For this review, take the finished solid that the model builds, in its own axes (mm). Face numbers are marked on the shaded views. A direction names the side the tool comes from. Coordinates: 2 decimals unless noted, no trailing zeros. Loops run counter-clockwise (first coordinate to the right, second up) from the corner with the lowest first, then second, coordinate; pieces in that order, holes last. Notation, with made-up numbers: M -38.75,19.5 L -9.75,19.5 A4 ccw -9.75,25.5 Z; hole C 62.25,21 d2. An arc over 180 degrees is marked long. Write item = value, one per line.
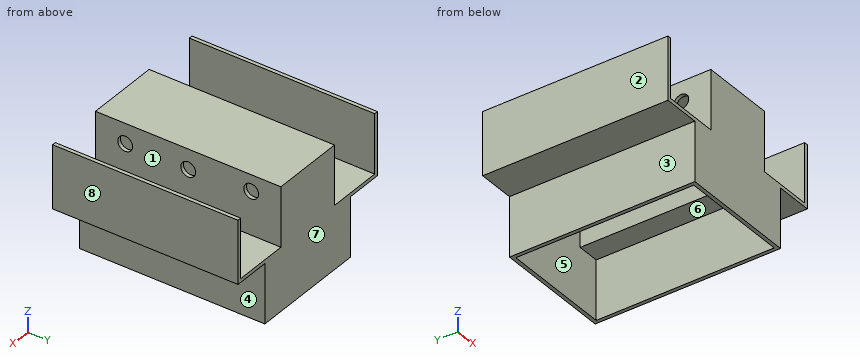
from build123d import *

# Parameters (mm, degrees)
ESQUISSE1_W             = 45
ESQUISSE1_H             = 250
BOSS_EXTRU_1_DEPTH      = 5
ESQUISSE2_W             = 80
ESQUISSE2_H             = 250
BOSS_EXTRU_2_DEPTH      = 5
ESQUISSE4_W             = 80
ESQUISSE4_H             = 250
BOSS_EXTRU_4_DEPTH      = 5
ESQUISSE5_W             = 85
ESQUISSE5_H             = 250
BOSS_EXTRU_5_DEPTH      = 5
ESQUISSE6_R             = 10
ENL_V_MAT_EXTRU_1_DEPTH = 5
ESQUISSE8_W             = 5
ESQUISSE8_H             = 250
BOSS_EXTRU_6_DEPTH      = 80
BOSS_EXTRU_7_DEPTH      = 5
BOSS_EXTRU_9_DEPTH      = 5


with BuildPart() as part:
    # Esquisse1 → Boss.-Extru.1 (new body)
    with BuildSketch(Plane.XY):
        with Locations((-22.5, 125)):
            Rectangle(ESQUISSE1_W, ESQUISSE1_H)
    boss_extru_1 = extrude(amount=BOSS_EXTRU_1_DEPTH)

    # Esquisse2 → Boss.-Extru.2 (add)
    with BuildSketch(Plane(origin=(0, 0, 0), x_dir=(0, 0, -1), z_dir=(1, 0, 0))):
        with Locations((35, 125)):
            Rectangle(ESQUISSE2_W, ESQUISSE2_H)
    boss_extru_2 = extrude(amount=BOSS_EXTRU_2_DEPTH)

    # Esquisse4 → Boss.-Extru.4 (add)
    with BuildSketch(Plane(origin=(0, 0, -75), x_dir=(-1, 0, 0), z_dir=(0, 0, -1))):
        with Locations((-40, 125)):
            Rectangle(ESQUISSE4_W, ESQUISSE4_H)
    boss_extru_4 = extrude(amount=BOSS_EXTRU_4_DEPTH)

    # Esquisse5 → Boss.-Extru.5 (add)
    with BuildSketch(Plane(origin=(80, 0, 0), x_dir=(0, 0, -1), z_dir=(1, 0, 0))):
        with Locations((37.5, 125)):
            Rectangle(ESQUISSE5_W, ESQUISSE5_H)
    boss_extru_5 = extrude(amount=BOSS_EXTRU_5_DEPTH)

    # Esquisse6 → Enlèv. mat.-Extru.1 (cut)
    with BuildSketch(Plane(origin=(5, 0, 0), x_dir=(0, 0, -1), z_dir=(1, 0, 0))):
        with Locations((22, 40)):
            Circle(ESQUISSE6_R)
        with Locations((22, 125)):
            Circle(ESQUISSE6_R)
        with Locations((17, 210)):
            Circle(ESQUISSE6_R)
    enl_v_mat_extru_1 = extrude(amount=-ENL_V_MAT_EXTRU_1_DEPTH, mode=Mode.SUBTRACT)

    # Esquisse8 → Boss.-Extru.6 (add)
    with BuildSketch(Plane(origin=(0, 0, -80), x_dir=(-1, 0, 0), z_dir=(0, 0, -1))):
        with Locations((-32.5, 125)):
            Rectangle(ESQUISSE8_W, ESQUISSE8_H)
    boss_extru_6 = extrude(amount=BOSS_EXTRU_6_DEPTH)

    # Symétrie2: Boss.-Extru.1, Boss.-Extru.2, Boss.-Extru.4, Boss.-Extru.5, Enlèv. mat.-Extru.1, Boss.-Extru.6 across plane
    add(boss_extru_1.mirror(Plane(origin=(-45, 0, 5), x_dir=(0, 0, 1), z_dir=(1, 0, 0))))
    add(boss_extru_2.mirror(Plane(origin=(-45, 0, 5), x_dir=(0, 0, 1), z_dir=(1, 0, 0))))
    add(boss_extru_4.mirror(Plane(origin=(-45, 0, 5), x_dir=(0, 0, 1), z_dir=(1, 0, 0))))
    add(boss_extru_5.mirror(Plane(origin=(-45, 0, 5), x_dir=(0, 0, 1), z_dir=(1, 0, 0))))
    add(enl_v_mat_extru_1.mirror(Plane(origin=(-45, 0, 5), x_dir=(0, 0, 1), z_dir=(1, 0, 0))), mode=Mode.SUBTRACT)
    add(boss_extru_6.mirror(Plane(origin=(-45, 0, 5), x_dir=(0, 0, 1), z_dir=(1, 0, 0))))

    # Esquisse3D1 → Boss.-Extru.7 (add)
    with BuildSketch(Plane(origin=(30, 0, -160), x_dir=(-0.5999999999999998, 0, 0.8000000000000003), z_dir=(0, -1, 0))):
        Polygon((0, 0), (64, -48), (82, -24), (146, -72), (200, 0), (136, 48), (154, 72), (90, 120), align=None)
    extrude(amount=-BOSS_EXTRU_7_DEPTH)

    # Esquisse3D3 → Boss.-Extru.9 (add)
    with BuildSketch(Plane(origin=(-120, 250, -160), x_dir=(0.5999999999999999, 0, 0.8), z_dir=(0, 1, 0))):
        Polygon((0, 0), (64, -48), (82, -24), (146, -72), (200, 0), (136, 48), (154, 72), (90, 120), align=None)
    extrude(amount=-BOSS_EXTRU_9_DEPTH)


solid = part.part
Q1. For line 1 along X through (y, z) = (189, -8); line 2 along Y through (x, z) = (-47, -129.5); line 3 along X through (y, z) = (166.5, -81.5), list the stretches that pass through material, from the lowest coordinate up.
Solved:
line_1 = -175 to -170, -95 to -90, 0 to 5, 80 to 85
line_2 = 0 to 5, 245 to 250
line_3 = -125 to -120, 30 to 35
Q2. For pin 1 Ø5 at (y, z) = (149.5, -142) entering from -X; pin 2 Ø9 at (x, y) = (-98, 178.5) entering from -Z; pin 3 Ø4 at (x, y) = (-26.5, 179.5) entering from -Z, all flat-tipped, find the tip position at first contact; note any pin that passes through.
Solved:
pin_1 = -125
pin_2 = -80
pin_3 = 0
Q3. Draft analysis for pull direction Y (two halves, no side actions). For the marked faces 6, 7 and 8, state which applies: +Y half, -Y half, draft (parallel to the pull), parting line (faces both ways), or undercut.
Solved:
face_6 = undercut
face_7 = +Y half
face_8 = draft
Q4. Add section B-B (z = -141). Write out the cut boundary in (x, y).
Solved:
outline = M -125,0 L 35,0 L 35,250 L -125,250 Z; hole M -120,5 L 30,5 L 30,245 L -120,245 Z
Q5. Machinability: for the marked faces 1, 2, 3, 4 and 5, which of the approach directions +Z, -Z, +X, -X, +Y, -Y give a long, thin tool a straight path to every point of the face, cutting with its end or side? Answer none if there is none.
Solved:
face_1 = +Z, +Y, -Y
face_2 = +Z, -Z, -X, +Y, -Y
face_3 = -Z, -X, +Y, -Y
face_4 = -Z, +X, +Y, -Y
face_5 = -Z
Q6. Add section A-A (y = 125). State how many separate pieces and enclosed holes the cut face has, and give its area (3 significant figures).
Solved:
separate_pieces = 3
enclosed_holes = 0
area = 3,500 mm²
Q7. Add section D-D (y = 60). Write out the cut boundary in (x, z), and give its area (3 significant figures).
Solved:
outline = M -175,-80 L -125,-80 L -125,-160 L -120,-160 L -120,-80 L -90,-80 L -90,0 L 0,0 L 0,-80 L 30,-80 L 30,-160 L 35,-160 L 35,-80 L 85,-80 L 85,5 L 80,5 L 80,-75 L 5,-75 L 5,5 L -95,5 L -95,-75 L -170,-75 L -170,5 L -175,5 Z
area = 3,700 mm²
Q8. Add section C-C (x = -112). Write out the cut boundary in (y, z), and give its area (3 significant figures).
Solved:
outline = M 0,-160 L 5,-160 L 5,-80 L 245,-80 L 245,-160 L 250,-160 L 250,-75 L 0,-75 Z
area = 2,050 mm²
